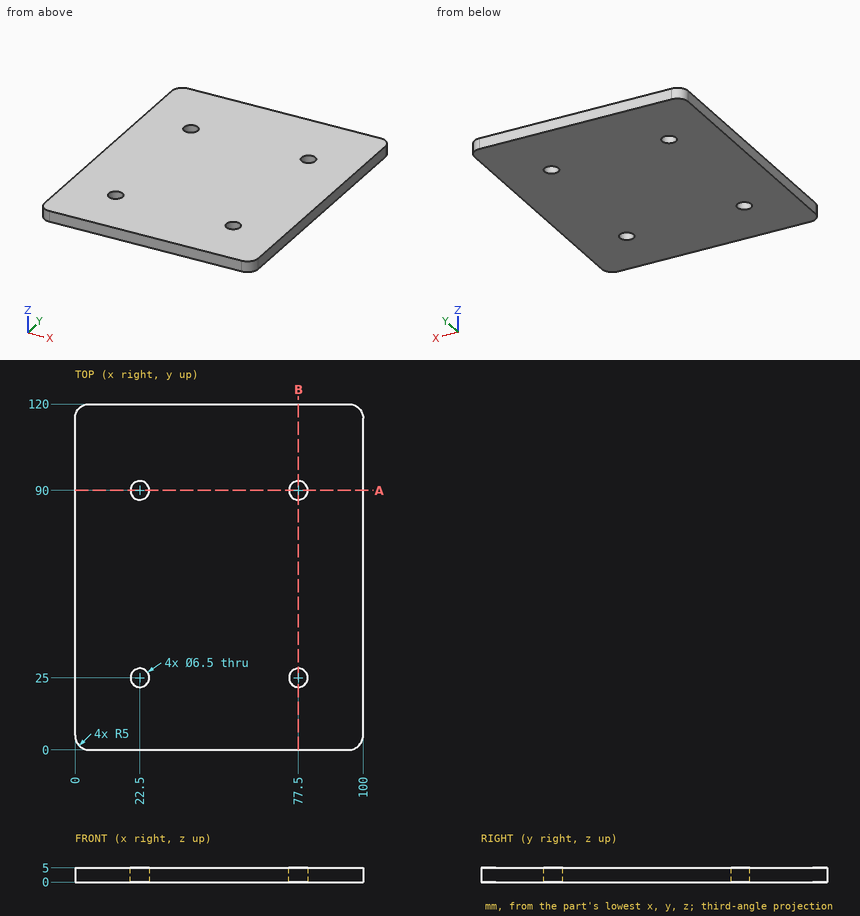
Design review of the part shown in the three views and the two pictorial views. Dimensions are in mm from the part's minimum x, y and z. Round coordinates to 2 decimals unless told otherwise and drop trailing zeros. Loops run counter-clockwise (first coordinate to the right, second up) from the corner with the lowest first, then second, coordinate; pieces in that order, holes last.
(1) We need section A-A (y = 90). Give the boundary of the cut face in (x, z), plus the area to 3 significant figures.
Returned:
outline: (0, 0) - (19.25, 0) - (19.25, 5) - (0, 5) - close; (25.75, 0) - (74.25, 0) - (74.25, 5) - (25.75, 5) - close; (80.75, 0) - (100, 0) - (100, 5) - (80.75, 5) - close
area: 435 mm2
(2) We need section B-B (x = 77.5). Give the boundary of the cut face in (y, z).
Returned:
outline: (0, 0) - (21.75, 0) - (21.75, 5) - (0, 5) - close; (28.25, 0) - (86.75, 0) - (86.75, 5) - (28.25, 5) - close; (93.25, 0) - (120, 0) - (120, 5) - (93.25, 5) - close
(3) Wall thickness on line 1 along Y through (x, z) = (77.5, 3.75); line 2 along Y through (x, z) = (20.5, 2.9); line 3 along Y through (x, z) = (96, 1.8): over which ranges is each line inside the solid? List them lowest first.
Returned:
line 1: y = 0 to 21.75, 28.25 to 86.75, 93.25 to 120
line 2: y = 0 to 22.44, 27.56 to 87.44, 92.56 to 120
line 3: y = 0.1 to 119.9
